Geometry: see drawing. Coordinates: mm, zero at the bounding-box minimum. A direction names the side the tool comes from. Coordinates: 2 decimals unless noted, no trailing zeros. Order: outer loops, then holes, each group sorted by start corner. A loop starts at its lowest first (then second) coordinate and runs counter-clockwise, first axis right, second up.
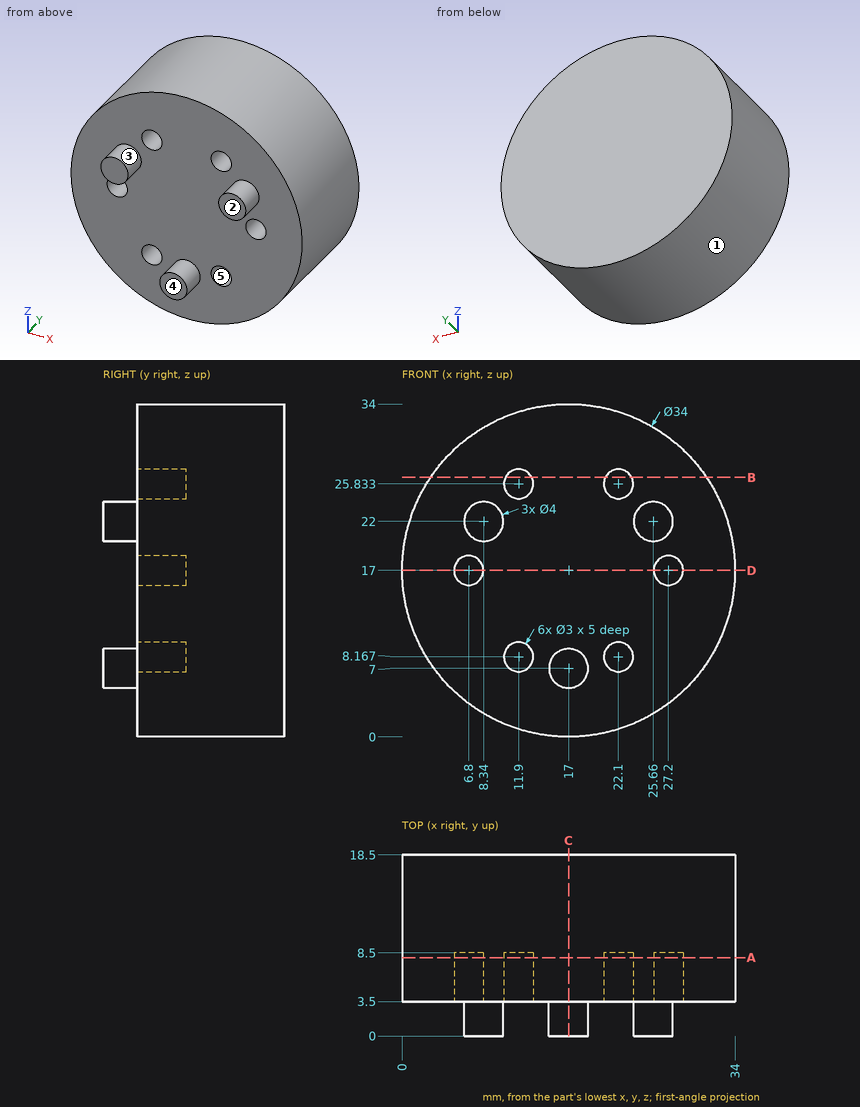
Item 1: Draft query along X for the marked faces 1, 2 and 3. Return one class per face: pulls with the +X half, pulls with the -X half, needs draft (parallel to the pull), parting line crosses it, or undercut.
Response values:
face 1: parting line crosses it
face 2: needs draft
face 3: undercut
Item 2: Access query for the marked faces 4 and 5. Directions: +Z, -Z, +X, -X, +Y, -Y. A direction counts if a zero-diameter tool reaches every point of the face in a straight line with its end or side. Return the directions, or none.
Response values:
face 4: +Z, -Z, +X, -X, -Y
face 5: -Y
Item 3: Cut plane A-A on y = 8. Return loops of the section in (x, z).
Response values:
outline: circle Ø34 at (17, 17); hole circle Ø3 at (6.8, 17); hole circle Ø3 at (11.9, 8.17); hole circle Ø3 at (11.9, 25.83); hole circle Ø3 at (22.1, 8.17); hole circle Ø3 at (22.1, 25.83); hole circle Ø3 at (27.2, 17)
Item 4: Cut plane B-B on z = 26.5. Return loops of the section in (x, y), then the cut area to 3 significant figures.
Response values:
outline: (2.9, 3.5) - (10.56, 3.5) - (10.56, 8.5) - (13.24, 8.5) - (13.24, 3.5) - (20.76, 3.5) - (20.76, 8.5) - (23.44, 8.5) - (23.44, 3.5) - (31.1, 3.5) - (31.1, 18.5) - (2.9, 18.5) - close
area: 396 mm2
Item 5: Pin query (flat end, axial travel): pin 1 Ø2.5 at (x, z) = (22.1, 8.17) entering from -Y; pin 2 Ø6 at (y, z) = (5, 24) entering from +X; pin 3 Ø3.5 at (x, z) = (11.5, 7.5) entering from -Y. Return the tip coordinate at first contact, or that it passes through.
Response values:
pin 1: stops at y = 8.5
pin 2: stops at x = 33.52
pin 3: stops at y = 3.5
Item 6: Ray query, probe 1 along X at (y, z) = (6.95, 17); probe 2 along Z at (x, y) = (11, 8) (1 decimal); probe 3 along Y at (x, z) = (12, 15.5). Return the intervals inside material, ascending.
Response values:
probe 1: x = 0 to 5.3, 8.3 to 25.7, 28.7 to 34
probe 2: z = 1.1 to 7, 9.4 to 24.6, 27 to 32.9
probe 3: y = 3.5 to 18.5
Item 7: Cut plane D-D on z = 17. Return loops of the section in (x, y), then the cut area to 3 significant figures.
Response values:
outline: (0, 3.5) - (5.3, 3.5) - (5.3, 8.5) - (8.3, 8.5) - (8.3, 3.5) - (25.7, 3.5) - (25.7, 8.5) - (28.7, 8.5) - (28.7, 3.5) - (34, 3.5) - (34, 18.5) - (0, 18.5) - close
area: 480 mm2
Item 8: Cut plane C-C on x = 17. Return loops of the section in (y, z).
Response values:
outline: (0, 5) - (3.5, 5) - (3.5, 0) - (18.5, 0) - (18.5, 34) - (3.5, 34) - (3.5, 9) - (0, 9) - close
